Design review of the part built by this model. Coordinates are the model's own, in mm. Face numbers are marked on the shaded views. A direction names the side the tool comes from. Coordinates: 2 decimals unless noted, no trailing zeros. Write each loop counter-clockwise with the first axis right and the second up, starting at its lowest first coordinate (ties: lowest second). Pieces come first, ordered by that corner, then holes.
Q1. Machinability: for the marked faces 1, 2 and 3, which of the approach directions +Z, -Z, +X, -X, +Y, -Y give a long, thin tool a straight path to every point of the face, cutting with its end or side? Answer none if there is none.
Q2. Add section B-B, the plane y = 7. Give the boundary of the cut face in (x, z), plus the area to 3 significant figures.
Q3. Add section A-A, the plane y = 49.5. Give the boundary of the cut face in (x, z).
Q4. Clearance check with flat-ended pins moving along their axes: pin 1 Ø5 at (y, z) = (24.5, -9.5) entering from +X; pin 2 Ø3 at (x, y) = (-4, 55.5) entering from -Z; pin 3 Ø1.5 at (x, z) = (9, 7) entering from +Y; pin 4 Ø12 at (y, z) = (27.5, 6) entering from +X. State where each tip first meets the part, or that it passes through.
Q5. To check wall thickness, follow probe 1 along X at (y, z) = (0.65, 0); probe 2 along Z at (x, y) = (6.5, 4); probe 3 along Z at (x, y) = (0, 78.5). State the ranges of each line that lie inside material, in increasing order.
from build123d import *

# Parameters (mm, degrees)
SKETCH1_R           = 15
BOSS_EXTRUDE1_DEPTH = 5
SKETCH2_R           = 5
BOSS_EXTRUDE2_DEPTH = 90
CUT_EXTRUDE1_START  = -15
CUT_EXTRUDE1_DEPTH  = 15
SKETCH4_W           = 2
SKETCH4_H           = 5.2
CUT_EXTRUDE2_DEPTH  = 99.17076958
FILLET1_R           = 10
FILLET2_R           = 2
CUT_EXTRUDE3_DEPTH  = 1
SKETCH6_R           = 13.5
SKETCH6_R_2         = 11.5
CUT_EXTRUDE4_DEPTH  = 1


with BuildPart() as part:
    # Sketch1 → Boss-Extrude1 (new body)
    with BuildSketch(Plane(origin=(0, 0, 0), x_dir=(1, 0, 0), z_dir=(0, 1, 0))):
        with Locations(Location((0, 0, 0), (0, 0, 270))):
            Circle(SKETCH1_R)
    extrude(amount=BOSS_EXTRUDE1_DEPTH)

    # Sketch2 → Boss-Extrude2 (add)
    with BuildSketch(Plane(origin=(0, 5, 0), x_dir=(1, 0, 0), z_dir=(0, 1, 0))):
        with Locations(Location((0, 0, 0), (0, 0, 90))):
            Circle(SKETCH2_R)
    extrude(amount=BOSS_EXTRUDE2_DEPTH)

    # Sketch3 → Cut-Extrude1 (cut)
    with BuildSketch(Plane(origin=(0, 95, 0), x_dir=(1, 0, 0), z_dir=(0, 1, 0)).offset(CUT_EXTRUDE1_START)):
        with BuildLine():
            Line((0, 5), (5, 0))
            ThreePointArc((5, 0), (3.535533906, 3.535533906), (0, 5))
        make_face()
    extrude(amount=CUT_EXTRUDE1_DEPTH, mode=Mode.SUBTRACT)

    # Sketch4 → Cut-Extrude2 (cut, through all)
    with BuildSketch(Plane(origin=(2.5, 0, -2.5), x_dir=(-0.7071067811865475, 0, -0.7071067811865477), z_dir=(0.7071067811865477, 0, -0.7071067811865475))):
        with Locations((0, 87.5)):
            Rectangle(SKETCH4_W, SKETCH4_H)
    extrude(amount=-CUT_EXTRUDE2_DEPTH, mode=Mode.SUBTRACT)

    # Fillet1
    fillet1_edges = [part.edges().sort_by_distance(p)[0] for p in [
        (0, 5, 5),
    ]]
    fillet(fillet1_edges, radius=FILLET1_R - 0.0001)  # a hair under: the kernel refuses the full size

    # Fillet2
    fillet2_edges = [part.edges().sort_by_distance(p)[0] for p in [
        (0, 5, -15),
    ]]
    fillet(fillet2_edges, radius=FILLET2_R)

    # Sketch5 → Cut-Extrude3 (cut)
    with BuildSketch(Plane.XZ):
        with BuildLine():
            Line((-1.637065711, 9.676642787), (9.523190699, -1.483613623))
            Line((9.523190699, -1.483613623), (5.311652237, -5.695152084))
            add(Edge.make_bspline(
                [(5.311652237, -5.695152084), (5.222138514, -5.784060594), (5.04738551, -5.957632072), (4.789980879, -6.205637327), (4.545170464, -6.434144406), (4.314659572, -6.644098006), (4.09362148, -6.830927906), (3.889758382, -7.002719589), (3.69565283, -7.150200035), (3.570345293, -7.241295339), (3.510370186, -7.284895674)],
                knots=[0, 0, 0, 0, 1.258886347, 2.457658598, 3.566401057, 4.600468819, 5.568286539, 6.454134328, 7.260112675, 8, 8, 8, 8], degree=3))
            add(Edge.make_bspline(
                [(3.510370186, -7.284895674), (3.352057488, -7.391657893), (3.045888719, -7.598130638), (2.566454347, -7.848616029), (2.088709315, -8.031605789), (1.611555846, -8.155041162), (1.129098311, -8.206051584), (0.637891361, -8.192108975), (0.134888923, -8.11428248), (-0.372633356, -7.969030769), (-0.872601546, -7.763082396), (-1.351797855, -7.491862034), (-1.809467136, -7.167166368), (-2.084445811, -6.906961882), (-2.223604173, -6.775280289)],
                knots=[0, 0, 0, 0, 1.085817505, 2.099916266, 3.069631314, 3.991048598, 4.895916369, 5.820176367, 6.779587027, 7.784039251, 8.816928408, 9.848367769, 10.911124231, 12, 12, 12, 12], degree=3))
            add(Edge.make_bspline(
                [(-2.223604173, -6.775280289), (-2.336734542, -6.656352184), (-2.56008707, -6.421553226), (-2.855775684, -6.042833727), (-3.106227984, -5.64686054), (-3.315994358, -5.238308237), (-3.484073648, -4.815633421), (-3.609745523, -4.377562245), (-3.691600055, -3.924500762), (-3.737830146, -3.456793519), (-3.718915595, -2.972046746), (-3.62400832, -2.471794707), (-3.445196287, -1.960272191), (-3.195874633, -1.431943292), (-2.869308405, -0.889700641), (-2.464234681, -0.334885684), (-1.986644206, 0.236940057), (-1.625835114, 0.606436234), (-1.438347763, 0.798437659)],
                knots=[0, 0, 0, 0, 0.905918046, 1.788547915, 2.647703894, 3.489284766, 4.320694788, 5.155279578, 6.001046779, 6.859817908, 7.745360365, 8.669757575, 9.660298499, 10.729041634, 11.890420876, 13.149445516, 14.5187654, 16, 16, 16, 16], degree=3))
            Line((-1.438347763, 0.798437659), (1.423831724, 3.660617146))
            Line((1.423831724, 3.660617146), (-3.114629814, 8.199078685))
            Line((-3.114629814, 8.199078685), (-1.637065711, 9.676642787))
        make_face()
        with BuildLine():
            Line((2.737934289, 2.346514582), (-0.146681096, -0.538100802))
            add(Edge.make_bspline(
                [(-0.146681096, -0.538100802), (-0.260313381, -0.65428127), (-0.479959168, -0.878852573), (-0.773260091, -1.224420889), (-1.027081256, -1.559053853), (-1.234921637, -1.885549874), (-1.405033378, -2.201516333), (-1.532005524, -2.509259236), (-1.61338181, -2.809868657), (-1.653183343, -3.102018529), (-1.651825971, -3.386261795), (-1.620270356, -3.663837107), (-1.554866401, -3.935764915), (-1.458636403, -4.202624086), (-1.328091019, -4.463959906), (-1.167765432, -4.721763246), (-0.971104209, -4.971210552), (-0.822117923, -5.127940531), (-0.74604007, -5.207972597)],
                knots=[0, 0, 0, 0, 1.445903498, 2.794862496, 4.030928865, 5.180949829, 6.23580341, 7.221038598, 8.136693834, 9.000005142, 9.836726991, 10.659941899, 11.480957457, 12.32010686, 13.179061295, 14.076063356, 15.017567502, 16, 16, 16, 16], degree=3))
            add(Edge.make_bspline(
                [(-0.74604007, -5.207972597), (-0.6293357, -5.316302566), (-0.402138795, -5.527196413), (-0.019259163, -5.776250817), (0.382841414, -5.956890263), (0.800723528, -6.060399706), (1.219698662, -6.102803811), (1.630125751, -6.06432865), (2.028390936, -5.964880448), (2.271917157, -5.841059549), (2.394985571, -5.778485418)],
                knots=[0, 0, 0, 0, 1.110082986, 2.161079462, 3.172912607, 4.173354109, 5.154591278, 6.098016453, 7.038813575, 8, 8, 8, 8], degree=3))
            add(Edge.make_bspline(
                [(2.394985571, -5.778485418), (2.438170358, -5.752446879), (2.531164584, -5.696375427), (2.67205046, -5.59014108), (2.83334386, -5.466586503), (3.006975281, -5.314717262), (3.201771433, -5.144293582), (3.410529337, -4.950105092), (3.637256703, -4.7334163), (3.791622967, -4.580044579), (3.872549673, -4.499639264)],
                knots=[0, 0, 0, 0, 0.617675747, 1.330104431, 2.160457084, 3.107811318, 4.156123608, 5.332972174, 6.601807352, 8, 8, 8, 8], degree=3))
            Line((3.872549673, -4.499639264), (6.728318904, -1.643870033))
            Line((6.728318904, -1.643870033), (2.737934289, 2.346514582))
        make_face(mode=Mode.SUBTRACT)
    extrude(amount=-CUT_EXTRUDE3_DEPTH, mode=Mode.SUBTRACT)

    # Sketch6 → Cut-Extrude4 (cut)
    with BuildSketch(Plane.XZ):
        with Locations(Location((0, 0, 0), (0, 0, 270))):
            Circle(SKETCH6_R)
        with Locations(Location((0, 0, 0), (0, 0, 270))):
            Circle(SKETCH6_R_2, mode=Mode.SUBTRACT)
    extrude(amount=-CUT_EXTRUDE4_DEPTH, mode=Mode.SUBTRACT)


solid = part.part
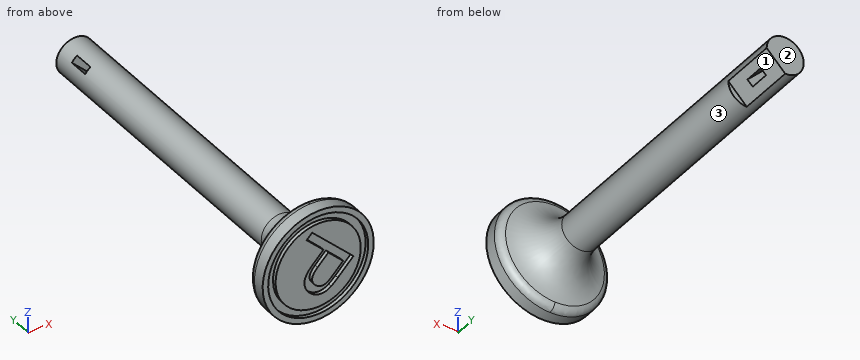
Here are the results:
1. face 1: -Z, +X, +Y
1. face 2: +Z, -Z, +X, -X, +Y
1. face 3: +Y
2. outline: circle Ø18 at (0, 0)
2. area: 254 mm2
3. outline: circle Ø10 at (0, 0)
4. pin 1: passes through
4. pin 2: stops at z = -4.33
4. pin 3: stops at y = 5.99
4. pin 4: stops at x = 5
5. probe 1: x = -15 to -13.5, -11.5 to -2.18, 0.39 to 5.08, 8.04 to 11.5, 13.5 to 15
5. probe 2: z = -13.32 to 13.32
5. probe 3: z = -5 to 5
